The listing builds one solid part. Answer for the finished solid, in the listing's coordinates (mm). A direction names the side the tool comes from. Coordinates: 2 decimals unless noted, no trailing zeros. Write each loop counter-clockwise with the first axis right and the second up, starting at its lowest first coordinate (ties: lowest second). Pieces come first, ordered by that corner, then holes.
from build123d import *

# Parameters (mm, degrees)
F0_W     = 13.5431550443
F0_H     = 2.539999783
F1_DEPTH = 14.478
F2_DEPTH = 25.4
F3_DEPTH = 15.24


with BuildPart() as f1:
    # F0 (on Front) → F1 (new body)
    with BuildSketch(Plane.XZ):
        with BuildLine():
            Line((-35.7278846204, 60.0338317454), (-46.2333224714, 60.0338317454))
            Line((-46.2333224714, 60.0338317454), (-46.2412260565, 53.5373517857))
            Line((-46.2412260565, 53.5373517857), (-62.0638123778, 53.5566014653))
            Line((-62.0638123778, 53.5566014653), (-62.0638123778, 28.5179335624))
            Line((-62.0638123778, 28.5179335624), (-46.2716645559, 28.5179335624))
            Line((-46.2716645559, 28.5179335624), (-46.2921659325, 11.6664945766))
            Line((-46.2921659325, 11.6664945766), (-60.9269401373, 11.6842991698))
            Line((-60.9269401373, 11.6842991698), (-60.9269401373, -11.473370716))
            Line((-60.9269401373, -11.473370716), (-60.9269401373, -12.8805553541))
            Line((-60.9269401373, -12.8805553541), (-60.9269401373, -22.7496541921))
            Line((-60.9269401373, -22.7496541921), (-46.3340580463, -22.7674078196))
            Line((-46.3340580463, -22.7674078196), (-23.9646863192, -22.7674078196))
            ThreePointArc((-23.9646863192, -22.7674078196), (-19.834707978, -21.8336374971), (-16.9685035944, -18.7169853598))
            Line((-16.9685035944, -18.7169853598), (-8.1312218681, 0))
            ThreePointArc((-8.1312218681, 0), (-3.0133196127, 1.4278545799), (0.6314046332, -2.4383680429))
            Line((0.6314046332, -2.4383680429), (25.4555270076, -49.4676344097))
            ThreePointArc((25.4555270076, -49.4676344097), (57.7549127304, -57.3994035782), (64.0637204051, -24.7442014515))
            Line((64.0637204051, -24.7442014515), (-5.2241440862, 57.5024038553))
            ThreePointArc((-5.2241440862, 57.5024038553), (-7.7229671621, 59.3967704345), (-10.7932919636, 60.0338317454))
            Line((-10.7932919636, 60.0338317454), (-22.1847295761, 60.0338317454))
            Line((-22.1847295761, 60.0338317454), (-22.1847295761, 49.3648834527))
            Line((-22.1847295761, 49.3648834527), (-22.1847295761, 46.8248836696))
            Line((-22.1847295761, 46.8248836696), (-22.1847295761, 44.971819967))
            Line((-22.1847295761, 44.971819967), (-35.7278846204, 44.971819967))
            Line((-35.7278846204, 44.971819967), (-35.7278846204, 46.8248836696))
            Line((-35.7278846204, 46.8248836696), (-35.7278846204, 49.3648834527))
            Line((-35.7278846204, 49.3648834527), (-35.7278846204, 60.0338317454))
        make_face()
        with BuildLine():
            Line((-27.5272410363, -17.2997955233), (-46.2700650096, -17.2997955233))
            Line((-46.2700650096, -17.2997955233), (-45.9628067911, 8.202736266))
            Line((-45.9628067911, 8.202736266), (-15.6977549195, 8.202736266))
            ThreePointArc((-15.6977549195, 8.202736266), (-12.7088773009, 6.3316862366), (-13.0860488862, 2.8256971855))
            Line((-13.0860488862, 2.8256971855), (-21.3820524514, -14.9953495711))
            ThreePointArc((-21.3820524514, -14.9953495711), (-24.1077143058, -17.0727256217), (-27.5272410363, -17.2997955233))
        make_face(mode=Mode.SUBTRACT)
        with Locations((-28.9563070983, 48.0948835611)):
            Rectangle(F0_W, F0_H)
    extrude(amount=F1_DEPTH)

    # F0 (on Front) → F2 (join)
    with BuildSketch(Plane.XZ):
        with BuildLine():
            Line((-35.7278846204, 60.0338317454), (-46.2333224714, 60.0338317454))
            Line((-46.2333224714, 60.0338317454), (-46.2412260565, 53.5373517857))
            Line((-46.2412260565, 53.5373517857), (-62.0638123778, 53.5566014653))
            Line((-62.0638123778, 53.5566014653), (-62.0638123778, 28.5179335624))
            Line((-62.0638123778, 28.5179335624), (-46.2716645559, 28.5179335624))
            Line((-46.2716645559, 28.5179335624), (-46.2921659325, 11.6664945766))
            Line((-46.2921659325, 11.6664945766), (-60.9269401373, 11.6842991698))
            Line((-60.9269401373, 11.6842991698), (-60.9269401373, -11.473370716))
            Line((-60.9269401373, -11.473370716), (-60.9269401373, -12.8805553541))
            Line((-60.9269401373, -12.8805553541), (-60.9269401373, -22.7496541921))
            Line((-60.9269401373, -22.7496541921), (-46.3340580463, -22.7674078196))
            Line((-46.3340580463, -22.7674078196), (-23.9646863192, -22.7674078196))
            ThreePointArc((-23.9646863192, -22.7674078196), (-19.834707978, -21.8336374971), (-16.9685035944, -18.7169853598))
            Line((-16.9685035944, -18.7169853598), (-8.1312218681, 0))
            ThreePointArc((-8.1312218681, 0), (-3.0133196127, 1.4278545799), (0.6314046332, -2.4383680429))
            Line((0.6314046332, -2.4383680429), (25.4555270076, -49.4676344097))
            ThreePointArc((25.4555270076, -49.4676344097), (57.7549127304, -57.3994035782), (64.0637204051, -24.7442014515))
            Line((64.0637204051, -24.7442014515), (-5.2241440862, 57.5024038553))
            ThreePointArc((-5.2241440862, 57.5024038553), (-7.7229671621, 59.3967704345), (-10.7932919636, 60.0338317454))
            Line((-10.7932919636, 60.0338317454), (-22.1847295761, 60.0338317454))
            Line((-22.1847295761, 60.0338317454), (-22.1847295761, 49.3648834527))
            Line((-22.1847295761, 49.3648834527), (-22.1847295761, 46.8248836696))
            Line((-22.1847295761, 46.8248836696), (-22.1847295761, 44.971819967))
            Line((-22.1847295761, 44.971819967), (-35.7278846204, 44.971819967))
            Line((-35.7278846204, 44.971819967), (-35.7278846204, 46.8248836696))
            Line((-35.7278846204, 46.8248836696), (-35.7278846204, 49.3648834527))
            Line((-35.7278846204, 49.3648834527), (-35.7278846204, 60.0338317454))
        make_face()
        with BuildLine():
            Line((-27.5272410363, -17.2997955233), (-46.2700650096, -17.2997955233))
            Line((-46.2700650096, -17.2997955233), (-45.9628067911, 8.202736266))
            Line((-45.9628067911, 8.202736266), (-15.6977549195, 8.202736266))
            ThreePointArc((-15.6977549195, 8.202736266), (-12.7088773009, 6.3316862366), (-13.0860488862, 2.8256971855))
            Line((-13.0860488862, 2.8256971855), (-21.3820524514, -14.9953495711))
            ThreePointArc((-21.3820524514, -14.9953495711), (-24.1077143058, -17.0727256217), (-27.5272410363, -17.2997955233))
        make_face(mode=Mode.SUBTRACT)
        with Locations((-28.9563070983, 48.0948835611)):
            Rectangle(F0_W, F0_H)
    extrude(amount=F2_DEPTH)

    # F0 (on Front) → F3 (join)
    with BuildSketch(Plane.XZ):
        with Locations((-28.9563070983, 48.0948835611)):
            Rectangle(F0_W, F0_H)
    extrude(amount=F3_DEPTH)


solid = f1.part
Q1. The part is cut by section B-B, the plane z = -53. Write down the section's boundary in (x, y).
Answers below:
outline: (27.94, -25.4) - (62.81, -25.4) - (62.81, 0) - (27.94, 0) - close
Q2. Which of the six approach directions +Z, -Z, +X, -X, +Y, -Y give full straight-line access (tool end or side, diameter ignored) to faces 1 (the face through (-29, -13, 49.365)), 2 (the face through (-12.61, -12.52, -9.49)), 3 (the face through (-17.176, -12.522, -5.96)), 4 (the face through (-60.927, -13, -5)), 5 (the face through (2, -25.4, 0))?
Answers below:
face 1: +Z, +Y, -Y
face 2: -Z, +Y, -Y
face 3: +Y, -Y
face 4: -Z, -X, +Y, -Y
face 5: +Z, -Z, +X, -X, -Y
Q3. Determine the mould class of faces 6 (the face through (-41, -13, 60.034)), 7 (the face through (-31, -13, 8.203)), 8 (the face through (29.905, -12.522, 15.803)) for opening direction X: released by +X, released by -X, zero draft, split by the parting line, or undercut.
Answers below:
face 6: zero draft
face 7: undercut
face 8: released by +X
Q4. The part is cut by section C-C, the plane x = 57. Write down the section's boundary in (y, z).
Answers below:
outline: (-25.4, -57.86) - (0, -57.86) - (0, -16.36) - (-25.4, -16.36) - close
Q5. Given pin 1 (12.5 mm diameter, centred on y = -11.5, z = -7, fed in from -X); pin 2 (3 mm diameter, centred on x = 6.5, z = 15.5, fed in from +Y); pin 3 (7.5 mm diameter, centred on x = -35.5, y = -18, fed in from -Z); pin 4 (12 mm diameter, centred on x = -1.5, y = -10.5, fed in from +Z), each flat-ended and moving along its own axis, determine where each tip first touches the part or whether it passes through.
Answers below:
pin 1: stops at x = -60.93
pin 2: stops at y = 0
pin 3: stops at z = -22.77
pin 4: stops at z = 59.29
Q6. Find the intervals of material crossed by probe 1 along Z at (x, y) = (-31, -8.5); probe 2 along Z at (x, y) = (-49, -2.5); probe 3 along X at (y, z) = (-21.5, 4), in increasing order.
Answers below:
probe 1: z = -22.77 to -17.3, 8.2 to 44.97, 46.82 to 49.36
probe 2: z = -22.76 to 11.67, 28.52 to 53.54
probe 3: x = -60.93 to -46.01, -12.49 to 39.85
Q7. The part is cut by section A-A, the plane y = -18.75. State how many separate pieces and enclosed holes the cut face has, then the cut area to 3 significant figures.
Answers below:
separate pieces: 1
enclosed holes: 2
area: 7,270 mm2
